Input: part model. Units: mm. Frame: model coordinates. A direction names the side the tool comes from. Give positions to 0.01 mm unless a question says otherwise; leave off trailing zeros. Loops run counter-clockwise (first coordinate to the right, second up) from the corner with the lowest first, then second, coordinate; pieces in that order, holes last. Notation, with made-up numbers: M -11.75,-1 L 10.25,-1 A34 ccw 10.25,30 Z; hole C -35.75,12.25 d2. An arc over 180 degrees is marked long. One line per item, written item: value. Start each with the question number.
(1) Pin query (flat end, axial travel): P1, Ø1.5, axis at x = -0.5, y = 2, coming from the -Z side; P2, Ø2, axis at x = -5, z = 3.5, coming from the -Y side; P3, Ø2, axis at x = 0, y = 2.5, coming from the +Z side; P4, Ø4, axis at x = 3, z = -2, coming from the +Y side. Return the tip coordinate at first contact, or that it passes through.
(2) Section C-C on y = -17. Output: boundary loops of the cut face in (x, z).
(3) Ray query, line 1 along Y through (x, z) = (3.5, -2); line 2 along X through (y, z) = (-18, 3); line 3 along Z through (x, y) = (0, 0.5). Return the intervals inside material, ascending. Write a range as from..to.
(4) Section B-B on z = -4. Output: boundary loops of the cut face in (x, y), plus the area to 3 significant figures.
(5) Access query for faces 1 (the cylindrical face through (-6, -17, 0)), 2 (the flat face through (0, 3, 1.1)), 3 (the flat face through (5, -9, 4)), 4 (the cylindrical face through (6, -17, 0)). Directions: +Z, -Z, +X, -X, +Y, -Y. A direction counts if a zero-diameter tool reaches every point of the face in a straight line with its end or side. Return the directions, or none.
(6) Section D-D on x = 2.25. Output: boundary loops of the cut face in (y, z), plus the area to 3 significant figures.
(7) Section A-A on x = 0. Output: boundary loops of the cut face in (y, z).
```python
from build123d import *

# Parameters (mm, degrees)
F0_W     = 12
F0_H     = 10
F1_DEPTH = 9
F3_DEPTH = 16.3
F5_DEPTH = 6


with BuildPart() as f1:
    # F0 (on Front) → F1 (new body)
    with BuildSketch(Plane.XZ):
        Rectangle(F0_W, F0_H)
    extrude(amount=F1_DEPTH)

    # F2 (on face) → F3 (join)
    with BuildSketch(Plane.XZ.offset(9)):
        with BuildLine():
            Line((3.316625, 5), (-3.316625, 5))
            ThreePointArc((-3.316625, 5), (-6, 0), (-3.316625, -5))
            Line((-3.316625, -5), (3.316625, -5))
            ThreePointArc((3.316625, -5), (6, 0), (3.316625, 5))
        make_face()
    extrude(amount=F3_DEPTH)

    # F4 (on face) → F5 (join)
    with BuildSketch(Plane(origin=(0, 0, 0), x_dir=(-1, 0, 0), z_dir=(0, 1, 0))):
        with BuildLine():
            Line((1.019804, 1.1), (-1.019804, 1.1))
            ThreePointArc((-1.019804, 1.1), (0, -1.5), (1.019804, 1.1))
        make_face()
    extrude(amount=F5_DEPTH)


solid = f1.part
```
Output values:
1. P1: stops at z = -1.5
1. P2: stops at y = -25.3
1. P3: stops at z = 1.1
1. P4: stops at y = 0
2. outline: M -3.32,-5 L 3.32,-5 A6 ccw 3.32,5 L -3.32,5 A6 ccw Z
3. line 1: y = -25.3..0
3. line 2: x = -5.2..5.2
3. line 3: z = -1.5..1.1
4. outline: M -6,-9 L -4.47,-9 L -4.47,-25.3 L 4.47,-25.3 L 4.47,-9 L 6,-9 L 6,0 L -6,0 Z
4. area: 254 mm²
5. face 1: -X, -Y
5. face 2: +Z, +X, -X, +Y
5. face 3: +Z, +X, -Y
5. face 4: +X, -Y
6. outline: M -25.3,-5 L 0,-5 L 0,5 L -25.3,5 Z
6. area: 253 mm²
7. outline: M -25.3,-5 L 0,-5 L 0,-1.5 L 6,-1.5 L 6,1.1 L 0,1.1 L 0,5 L -25.3,5 Z
